Part print with two shaded views. Sizes in mm from the minimum x, y, z corner. Round coordinates to 2 decimals unless told otherwise and drop trailing zeros. Write each loop counter-clockwise with the first axis right and the second up, starting at its lowest first coordinate (ties: lowest second). Pieces come first, ordered by that corner, then holes. Notation, with made-up numbers: (60, 74.5) -> (91, 74.5) arc R32 ccw to (91, 110.5) -> close; hole circle Ø9 at (64.5, -3.75). An arc over 180 degrees is marked (long way). Return JSON: item names as keys, results as strings. Group by question number.
(1) Saw through at B-B (z = 0.85). List the corners of the cut face in (x, y), plus the area to 3 significant figures.
(2) Saw through at D-D (y = 7). List the corners of the cut face in (x, z), plus the area to 3 significant figures.
(3) Drill centre lines: L1, parallel to Y at x = 7.5, z = 1; L2, parallel to X at y = 6, z = 0.5; L3, parallel to Y at x = 8.25, z = 1. Where is each one in solid material? Low to high. Write a range as from..to.
(4) Saw through at C-C (x = 7.5). List the corners of the cut face in (y, z).
(5) Saw through at A-A (y = 22). List the corners of the cut face in (x, z), plus the area to 3 significant figures.
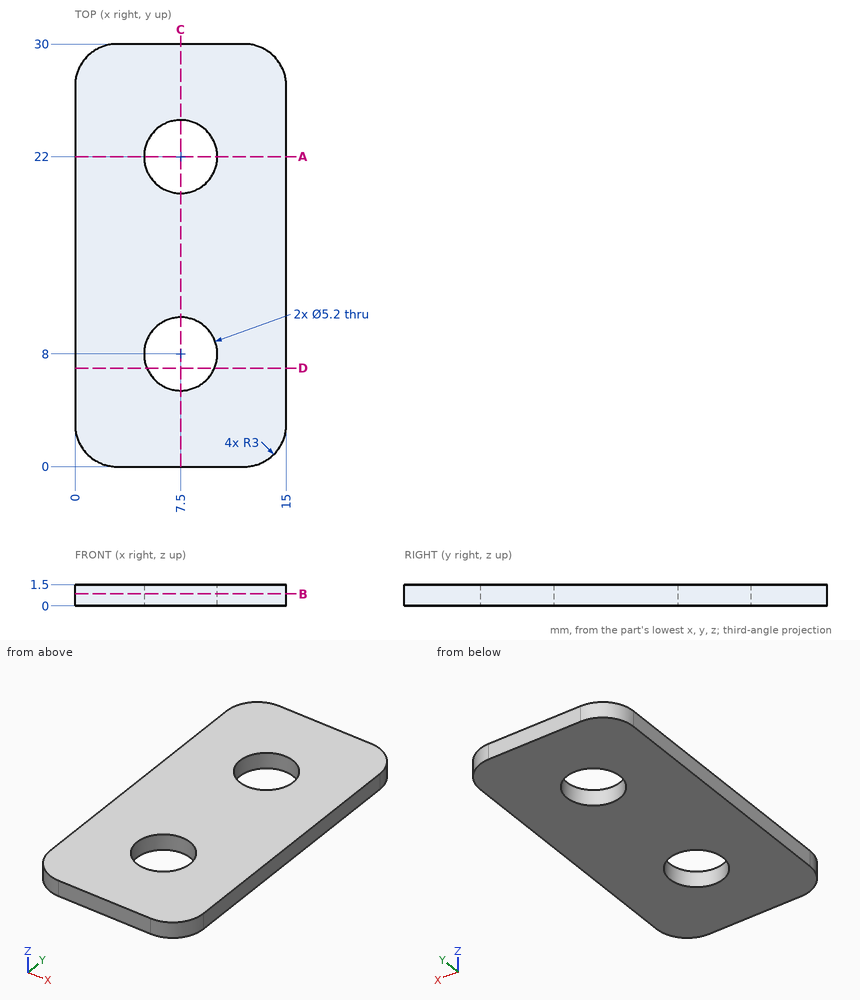
Computed values:
{
 "1": {"outline": "(0, 3) arc R3 ccw to (3, 0) -> (12, 0) arc R3 ccw to (15, 3) -> (15, 27) arc R3 ccw to (12, 30) -> (3, 30) arc R3 ccw to (0, 27) -> close; hole circle Ø5.2 at (7.5, 8); hole circle Ø5.2 at (7.5, 22)", "area": "400 mm2"},
 "2": {"outline": "(0, 0) -> (5.1, 0) -> (5.1, 1.5) -> (0, 1.5) -> close; (9.9, 0) -> (15, 0) -> (15, 1.5) -> (9.9, 1.5) -> close", "area": "15.3 mm2"},
 "3": {"L1": "0..5.4, 10.6..19.4, 24.6..30", "L2": "0..5.84, 9.16..15", "L3": "0..5.51, 10.49..19.51, 24.49..30"},
 "4": {"outline": "(0, 0) -> (5.4, 0) -> (5.4, 1.5) -> (0, 1.5) -> close; (10.6, 0) -> (19.4, 0) -> (19.4, 1.5) -> (10.6, 1.5) -> close; (24.6, 0) -> (30, 0) -> (30, 1.5) -> (24.6, 1.5) -> close"},
 "5": {"outline": "(0, 0) -> (4.9, 0) -> (4.9, 1.5) -> (0, 1.5) -> close; (10.1, 0) -> (15, 0) -> (15, 1.5) -> (10.1, 1.5) -> close", "area": "14.7 mm2"}
}
